Check sheet for the modelled part. Datum: model origin and axes. Units: mm. Face numbers are marked on the shaded views. A direction names the side the tool comes from. Give positions to 0.01 mm unless a question says otherwise; leave off trailing zeros. Order: outer loops, then holes, each group sorted by start corner. A loop starts at its lowest first (then second) coordinate and runs counter-clockwise, first axis right, second up.
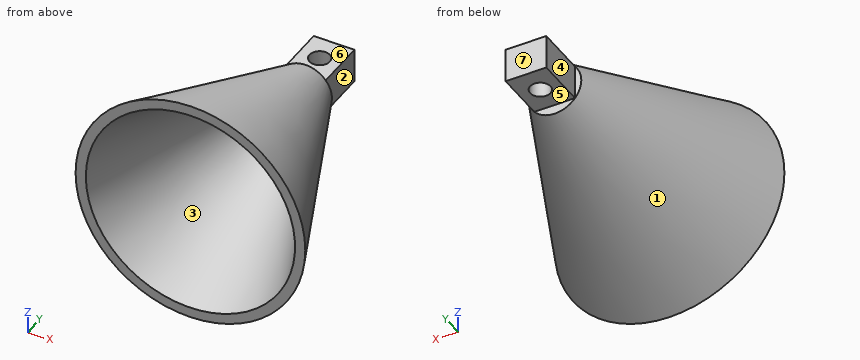
```python
from build123d import *

# Parameters (mm, degrees)
ESQUISSE2_W                  = 7.975229024
ESQUISSE2_H                  = 6.721241558
BOSS_EXTRU_1_DEPTH           = 10
ENL_V_MAT_EXTRU_1_DEPTH      = 14
ENL_V_MAT_EXTRU_1_DEPTH_BACK = 13


with BuildPart() as part:
    # Esquisse1 → Révolution1 (revolve)
    with BuildSketch(Plane.XY):
        Polygon((17.285132647, 40), (19.285132647, 40), (2, 0), (0, 0), align=None)
        Polygon((19.285132647, 40), (18.145144725, 37.361922653), (22.5, 37.361922653), (22.5, 40), align=None)
    revolve(axis=Axis((22.5, 40, 0), (0, -1, 0)))

    # Esquisse2 → Boss.-Extru.1 (add)
    with BuildSketch(Plane(origin=(0, 40, 0), x_dir=(1, 0, 0), z_dir=(0, 1, 0))):
        with Locations((22.5, 0)):
            Rectangle(ESQUISSE2_W, ESQUISSE2_H)
    extrude(amount=BOSS_EXTRU_1_DEPTH)

    # Esquisse3 → Enlèv. mat.-Extru.1 (cut, two sides)
    with BuildSketch(Plane(origin=(0, 0, -3.360620779), x_dir=(-1, 0, 0), z_dir=(0, 0, -1))) as enl_v_mat_extru_1_sk:
        with BuildLine():
            ThreePointArc((-20.5, 45), (-22.5, 47), (-24.5, 45))
            Line((-24.5, 45), (-20.5, 45))
        make_face()
        with BuildLine():
            Line((-20.5, 45), (-24.5, 45))
            ThreePointArc((-24.5, 45), (-22.5, 43), (-20.5, 45))
        make_face()
    extrude(amount=ENL_V_MAT_EXTRU_1_DEPTH, mode=Mode.SUBTRACT)
    extrude(enl_v_mat_extru_1_sk.sketch, amount=-ENL_V_MAT_EXTRU_1_DEPTH_BACK, mode=Mode.SUBTRACT)


solid = part.part
```
(1) Cross-section at C-C on x = 22.5. Enter the section's corners in (y, z).
Response values:
outline: (0, -22.5) - (40, -5.21) - (40, -3.36) - (43, -3.36) - (43, 3.36) - (40, 3.36) - (40, 5.21) - (0, 22.5) - (0, 20.5) - (37.36, 4.35) - (37.36, -4.35) - (0, -20.5) - close; (47, -3.36) - (50, -3.36) - (50, 3.36) - (47, 3.36) - close
(2) Set-up check for the marked faces 4, 5, 6 and 7: record each of +Z, -Z, +X, -X, +Y, -Y from which the full face is reachable in a straight line by a thin tool's end or side.
Response values:
face 4: +Z, -Z, -X, +Y
face 5: -Z, +X, -X, +Y
face 6: +Z, +X, -X, +Y
face 7: +Z, -Z, +X, -X, +Y
(3) Material ranges on L1, parallel to Y at x = 22.5, z = -1.25; L2, parallel to X at y = 45, z = -1.5; L3, parallel to X at y = 16, z = -6, recorded low to high.
Response values:
L1: y = 37.36 to 43, 47 to 50
L2: x = 18.51 to 20.5, 24.5 to 26.49
L3: x = 8.12 to 10.31, 34.69 to 36.88
(4) Cross-section at A-A on z = 0. Enter the section's corners in (x, y), then the cut area to 3 significant figures.
Response values:
outline: (0, 0) - (2, 0) - (18.15, 37.36) - (26.85, 37.36) - (43, 0) - (45, 0) - (27.71, 40) - (26.49, 40) - (26.49, 50) - (18.51, 50) - (18.51, 40) - (17.29, 40) - close; hole circle Ø4 at (22.5, 45)
area: 247 mm2
(5) Cross-section at B-B on y = 45. Enter the section's corners in (x, z).
Response values:
outline: (18.51, -3.36) - (20.5, -3.36) - (20.5, 3.36) - (18.51, 3.36) - close; (24.5, -3.36) - (26.49, -3.36) - (26.49, 3.36) - (24.5, 3.36) - close
(6) Release check for a two-part mould opening along Z. For the marked faces 1, 2 and 3 record: released by +Z, released by -Z, zero draft, split by the parting line, or undercut.
Response values:
face 1: split by the parting line
face 2: zero draft
face 3: undercut
(7) Cross-section at D-D on y = 30.5. Enter the section's corners in (x, z), then the cut area to 3 significant figures.
Response values:
outline: circle Ø18.64 at (22.5, 0); hole circle Ø14.64 at (22.5, 0)
area: 105 mm2
(8) Gauge pin test, flat ends, axial feed: pin 1 Ø6 at (x, z) = (40, 16.5) entering from +Y; pin 2 Ø3.5 at (y, z) = (46, 1.5) entering from -X; pin 3 Ø8 at (x, z) = (18.5, 8.5) entering from +Y; pin 4 Ø3.5 at (x, y) = (22.5, 45) entering from -Z. Record the tip position at first contact, or that the pin passes through.
Response values:
pin 1: stops at y = 3.35
pin 2: stops at x = 18.51
pin 3: stops at y = 39.59
pin 4: passes through
